The listing builds one solid part. Answer for the finished solid, in the listing's coordinates (mm). A direction names the side the tool comes from. Give positions to 0.01 mm unless a question says otherwise; leave off trailing zeros. Loops run counter-clockwise (first coordinate to the right, second up) from the corner with the lowest first, then second, coordinate; pieces in that order, holes last. Notation, with made-up numbers: (89, 61.5) -> (147, 61.5) arc R24 cw to (147, 91.5) -> close; hole circle Ø3 at (-7, -20). An arc over 180 degrees is marked (long way). One line per question, with ' | ' between items. Start each with the question number.
from build123d import *

# Parameters (mm, degrees)
M3X0_5_TAPPED_HOLE1_D     = 2.5
M3X0_5_TAPPED_HOLE1_DEPTH = 13.4874
M3X0_5_TAPPED_HOLE1_TIP   = 0.751075774
CUT_EXTRUDE1_REACH        = 185.602
SKETCH7_W                 = 50.8
SKETCH7_H                 = 2.565921067
CUT_EXTRUDE2_REACH        = 185.602
FILLET1_R                 = 1.5875
CIRPATTERN1_COUNT         = 9
FILLET1_OF_CIRPATTERN1_R  = 1.5875
SKETCH11_R                = 94
SKETCH11_R_2              = 90
CUT_EXTRUDE3_DEPTH        = 3


with BuildPart() as part:
    # Sketch1 → Revolve1 (revolve)
    with BuildSketch(Plane.XY, mode=Mode.PRIVATE) as revolve1_sk:
        Polygon((80.3783, 0), (127, 0), (127, 6.35), (98.425, 6.35), (98.425, 20.32), (110, 20.32), (110, 38.1), (102, 38.1), (102, 32.34), (80.3783, 32.34), align=None)
    revolve(revolve1_sk.sketch.rotate(Axis((0, 0, 0), (0, 1, 0)), 90), axis=Axis((0, 0, 0), (0, 1, 0)))

    # M3x0.5 Tapped Hole1
    with Locations(Plane(origin=(0, 38.1, 0), x_dir=(1, 0, 0), z_dir=(0, 1, 0))):
        with Locations((0, 105), (52.5, 90.932667397), (90.932667397, 52.5), (105, 0), (90.932667397, -52.5), (52.5, -90.932667397), (0, -105), (-52.5, -90.932667397), (-90.932667397, -52.5), (-105, 0), (-90.932667397, 52.5), (-52.5, 90.932667397)):
            Hole(M3X0_5_TAPPED_HOLE1_D / 2, depth=M3X0_5_TAPPED_HOLE1_DEPTH)
            with Locations((0, 0, -(M3X0_5_TAPPED_HOLE1_DEPTH + M3X0_5_TAPPED_HOLE1_TIP / 2))):  # 118° drill point
                Cone(0, M3X0_5_TAPPED_HOLE1_D / 2, M3X0_5_TAPPED_HOLE1_TIP, mode=Mode.SUBTRACT)

    # Sketch7 → Cut-Extrude1 (cut, up to next)
    with BuildSketch(Plane(origin=(0, 0, 0), x_dir=(1, 0, 0), z_dir=(0, 1, 0)), mode=Mode.PRIVATE) as cut_extrude1_sk1:
        with Locations((0, -125.717039467)):
            Rectangle(SKETCH7_W, SKETCH7_H)
    cut_extrude1_tool1 = extrude(cut_extrude1_sk1.sketch, amount=CUT_EXTRUDE1_REACH, mode=Mode.PRIVATE) & part.part
    add(cut_extrude1_tool1.solids().sort_by_distance((0, 0, 125.717039))[0], mode=Mode.SUBTRACT)

    # Sketch10 → Cut-Extrude2 (cut, up to next)
    with BuildSketch(Plane.XZ, mode=Mode.PRIVATE) as cut_extrude2_sk1:
        with BuildLine():
            Line((-3.3782, -106.045), (-3.3782, -127))
            Line((-3.3782, -127), (3.3782, -127))
            Line((3.3782, -127), (3.3782, -106.045))
            ThreePointArc((3.3782, -106.045), (0, -102.6668), (-3.3782, -106.045))
        make_face()
    cut_extrude2_tool1 = extrude(cut_extrude2_sk1.sketch, amount=-CUT_EXTRUDE2_REACH, mode=Mode.PRIVATE) & part.part
    cut_extrude2 = cut_extrude2_tool1.solids().sort_by_distance((0, 0, -115.183843))[0]
    add(cut_extrude2, mode=Mode.SUBTRACT)

    # Fillet1
    fillet1_edges = [part.edges().sort_by_distance(p)[0] for p in [
        (-3.3782, 3.175, -126.95506199),
        (3.3782, 3.175, -126.95506199),
    ]]
    fillet(fillet1_edges, radius=FILLET1_R)

    # CirPattern1: Cut-Extrude2 ×9 about axis
    cirpattern1_axis = Axis((0, 0, 0), (0, 1, 0))
    for i in range(1, CIRPATTERN1_COUNT):
        add(cut_extrude2.rotate(cirpattern1_axis, i * 360 / CIRPATTERN1_COUNT), mode=Mode.SUBTRACT)

    # Fillet1 of CirPattern1
    fillet1_of_cirpattern1_edges = [part.edges().sort_by_distance(p)[0] for p in [
        (-84.192992172, 3.175, -95.08175466),
        (-79.017289496, 3.175, -99.424684866),
        (-125.612947605, 3.175, -18.718637609),
        (-124.439711058, 3.175, -25.372392711),
        (-108.257208822, 3.175, 66.403138014),
        (-111.635408822, 3.175, 60.551923976),
        (-40.246718886, 3.175, 120.454147371),
        (-46.595658109, 3.175, 118.143322475),
        (46.595658109, 3.175, 118.143322475),
        (40.246718886, 3.175, 120.454147371),
        (111.635408822, 3.175, 60.551923976),
        (108.257208822, 3.175, 66.403138014),
        (124.439711058, 3.175, -25.372392711),
        (125.612947605, 3.175, -18.718637609),
        (79.017289496, 3.175, -99.424684866),
        (84.192992172, 3.175, -95.08175466),
    ]]
    fillet(fillet1_of_cirpattern1_edges, radius=FILLET1_OF_CIRPATTERN1_R)

    # Sketch11 → Cut-Extrude3 (cut)
    with BuildSketch(Plane(origin=(0, 32.34, 0), x_dir=(1, 0, 0), z_dir=(0, 1, 0))):
        with Locations(Location((0, 0, 0), (0, 0, 270))):
            Circle(SKETCH11_R)
        with Locations(Location((0, 0, 0), (0, 0, 270))):
            Circle(SKETCH11_R_2, mode=Mode.SUBTRACT)
    extrude(amount=-CUT_EXTRUDE3_DEPTH, mode=Mode.SUBTRACT)


solid = part.part
1. Straight lines are drawn through the part: L1, parallel to Y at x = 56.5, z = 90.5; L2, parallel to Z at x = -68, y = 32; L3, parallel to Y at x = -41, z = -90. For each, find the intervals that lie inside material, in ascending order.
2. The part is cut by section A-A (z = 13). Write down the section's boundary in (x, y), plus the area to 3 significant figures.
3. Each of these flat-tipped pins is pushed along its axis until it touches: pin 1 Ø8 at (y, z) = (29.5, 73) entering from -X; pin 2 Ø1.5 at (x, z) = (-90.93, 52.5) entering from -Y; pin 3 Ø3 at (y, z) = (2.5, -118.5) entering from -X. Where does it stop, or does it pass through?
4. Determine the mould class of faces 6 (the cylindrical face through (81.21, 3.22, 97.64)), 7 (the flat face through (-2, 0, 81)), 8 (the flat face through (-36.344, 3.131, 109.732)), 9 (the flat face through (-76.86, 3.13, -86.34)) for opening direction Z: released by +Z, released by -Z, zero draft, split by the parting line, or undercut.
5. For faces 1 (the flat face through (-3.378, 3, -116)), 2 (the flat face through (-38, 6.35, 92)), 3 (the cylindrical face through (-88.95, 3.13, 51.27)), 4 (the flat face through (0, 3, 124.434)), 5 (the cylindrical face through (63.53, 30.86, -69.28)), determine the directions among +Z, -Z, +X, -X, +Y, -Y from which every point of the face is accessible in a straight line to the end or side of a thin tool.
6. The part is cut by section B-B (z = -72). Write down the section's boundary in (x, y).
Check sheet entries:
1) L1: y = 0 to 6.35, 20.32 to 38.1 | L2: z = -86.46 to -64.9, -58.96 to -42.86, 42.86 to 58.96, 64.9 to 86.46 | L3: y = 0 to 6.35, 20.32 to 32.34
2) outline: (-126.33, 0) -> (-79.32, 0) -> (-79.32, 32.34) -> (-89.06, 32.34) -> (-89.06, 29.34) -> (-93.1, 29.34) -> (-93.1, 32.34) -> (-101.17, 32.34) -> (-101.17, 38.1) -> (-109.23, 38.1) -> (-109.23, 20.32) -> (-97.56, 20.32) -> (-97.56, 6.35) -> (-126.33, 6.35) -> close; (79.32, 0) -> (126.33, 0) -> (126.33, 6.35) -> (97.56, 6.35) -> (97.56, 20.32) -> (109.23, 20.32) -> (109.23, 38.1) -> (101.17, 38.1) -> (101.17, 32.34) -> (93.1, 32.34) -> (93.1, 29.34) -> (89.06, 29.34) -> (89.06, 32.34) -> (79.32, 32.34) -> close | area: 1,890 mm^2
3) pin 1: stops at x = -85.67 | pin 2: stops at y = 20.32 | pin 3: stops at x = -49.4
4) face 6: released by +Z | face 7: zero draft | face 8: undercut | face 9: undercut
5) face 1: -Z, -Y | face 2: none | face 3: -Y | face 4: +Z, +X, -X, +Y, -Y | face 5: +Y
6) outline: (-104.62, 0) -> (-35.73, 0) -> (-35.73, 32.34) -> (-54, 32.34) -> (-54, 29.34) -> (-60.43, 29.34) -> (-60.43, 32.34) -> (-72.25, 32.34) -> (-72.25, 38.1) -> (-83.16, 38.1) -> (-83.16, 20.32) -> (-67.11, 20.32) -> (-67.11, 6.35) -> (-104.62, 6.35) -> close; (35.73, 0) -> (104.62, 0) -> (104.62, 6.35) -> (67.11, 6.35) -> (67.11, 20.32) -> (83.16, 20.32) -> (83.16, 38.1) -> (72.25, 38.1) -> (72.25, 32.34) -> (60.43, 32.34) -> (60.43, 29.34) -> (54, 29.34) -> (54, 32.34) -> (35.73, 32.34) -> close
